from build123d import *

# Parameters (mm, degrees)
SKETCH1_R           = 19
SKETCH1_R_2         = 1
BOSS_EXTRUDE1_DEPTH = 1.6
SKETCH2_W           = 16.970562748
SKETCH2_H           = 3.563360777
SKETCH2_W_2         = 5.149879678
SKETCH2_H_2         = 16.970562749
CUT_EXTRUDE1_DEPTH  = 1.6
CUT_EXTRUDE2_DEPTH  = 1.6
SKETCH4_W           = 16
SKETCH4_H           = 11.067837439
CUT_EXTRUDE3_DEPTH  = 1.6


with BuildPart() as part:
    # Sketch1 → Boss-Extrude1 (new body)
    with BuildSketch(Plane.XY):
        with Locations((0, -13.250389013)):
            Circle(SKETCH1_R)
        with Locations((-10, -3.250389013)):
            Circle(SKETCH1_R_2, mode=Mode.SUBTRACT)
        with Locations((10, -3.250389013)):
            Circle(SKETCH1_R_2, mode=Mode.SUBTRACT)
        with Locations((10, -23.250389013)):
            Circle(SKETCH1_R_2, mode=Mode.SUBTRACT)
        with Locations((-10, -23.250389013)):
            Circle(SKETCH1_R_2, mode=Mode.SUBTRACT)
    extrude(amount=BOSS_EXTRUDE1_DEPTH)

    # Sketch2 → Cut-Extrude1 (cut)
    with BuildSketch(Plane.XY.offset(1.6)):
        with Locations((0, 5.531291376)):
            Rectangle(SKETCH2_W, SKETCH2_H)
        with Locations((-19.574939839, -13.250389013)):
            Rectangle(SKETCH2_W_2, SKETCH2_H_2)
    extrude(amount=-CUT_EXTRUDE1_DEPTH, mode=Mode.SUBTRACT)

    # Sketch3 → Cut-Extrude2 (cut)
    with BuildSketch(Plane(origin=(0, 0, 0), x_dir=(-1, 0, 0), z_dir=(0, 0, -1))):
        Polygon((12.5, -5.150389013), (12.5, -7.050389013), (17, -7.050389013), (24.21815824, -7.050389013), (24.21815824, 1.058699009), (18.989854596, 1.058699009), (12.5, 1.058699009), align=None)
    cut_extrude2 = extrude(amount=-CUT_EXTRUDE2_DEPTH, mode=Mode.SUBTRACT)

    # Mirror1: Cut-Extrude2 across plane
    add(cut_extrude2.mirror(Plane(origin=(0, 0, 0), x_dir=(0, 0, 1), z_dir=(1, 0, 0))), mode=Mode.SUBTRACT)

    # Sketch4 → Cut-Extrude3 (cut)
    with BuildSketch(Plane.XY.offset(1.6)):
        with Locations((0, -31.284307733)):
            Rectangle(SKETCH4_W, SKETCH4_H)
    extrude(amount=-CUT_EXTRUDE3_DEPTH, mode=Mode.SUBTRACT)


solid = part.part
Here's how the part is built. I have some questions about the finished solid (model axes, mm). A direction names the side the tool comes from. Coordinates: 2 decimals unless noted, no trailing zeros. Order: outer loops, then holes, each group sorted by start corner. A loop starts at its lowest first (then second) coordinate and runs counter-clockwise, first axis right, second up.
Item 1: For P1, Ø0.5, axis at y = -27.5, z = 1, coming from the -X side, with a flat end and sliding along its axis, tell me the tip position at first contact or that it passes through.
Result sheet:
P1: stops at x = -12.85
Item 2: I need wall thicknesses on line 1 (Y direction, x = 10, z = 1.1); line 2 (X direction, y = -4, z = 0.2); line 3 (Y direction, x = -6, z = 1.4). Which ranges of each line are inside material? Lowest first, please.
Result sheet:
line 1: y = -29.41 to -24.25, -22.25 to -4.25, -2.25 to 2.91
line 2: x = -12.5 to -10.66, -9.34 to 9.34, 10.66 to 12.5
line 3: y = -25.75 to 3.75
Item 3: If we section it at A-A on x = 10: List the corners of the cut face in (y, z) for me, plus the area to 3 significant figures.
Result sheet:
outline: (-29.41, 0) - (-24.25, 0) - (-24.25, 1.6) - (-29.41, 1.6) - close; (-22.25, 0) - (-4.25, 0) - (-4.25, 1.6) - (-22.25, 1.6) - close; (-2.25, 0) - (2.91, 0) - (2.91, 1.6) - (-2.25, 1.6) - close
area: 45.3 mm2
Item 4: For faces 5 (the face through (12.5, -3, 1)), 6 (the face through (-17, -14, 1)), 7 (the face through (8, -28, 1)), 8 (the face through (0, 3.75, 1)), 9 (the face through (-15, -7.05, 1)), which set-ups out of +Z, -Z, +X, -X, +Y, -Y let a thin tool reach every point of the face, with its end or its side?
Result sheet:
face 5: +Z, -Z, +X, +Y
face 6: +Z, -Z, -X, +Y, -Y
face 7: +Z, -Z, -Y
face 8: +Z, -Z, +X, -X, +Y
face 9: +Z, -Z, -X, +Y
Item 5: If we section it at C-C on x = 3.5: List the corners of the cut face in (y, z) for me, plus the area to 3 significant figures.
Result sheet:
outline: (-25.75, 0) - (3.75, 0) - (3.75, 1.6) - (-25.75, 1.6) - close
area: 47.2 mm2
Item 6: If we section it at D-D on y = -1: List the corners of the cut face in (x, z) for me, plus the area to 3 significant figures.
Result sheet:
outline: (-12.5, 0) - (12.5, 0) - (12.5, 1.6) - (-12.5, 1.6) - close
area: 40.0 mm2
Item 7: If we mould it in two halves opening along X, with no side actions, what happens to faces 1 (the face through (15, -7.05, 1)), 2 (the face through (-10.794, -3.859, 0.789)), 3 (the face through (0, -25.75, 1)), 4 (the face through (17.41, -20.86, 0.79))? For each: +X half, -X half, draft (parallel to the pull), parting line (faces both ways), or undercut.
Result sheet:
face 1: draft
face 2: undercut
face 3: undercut
face 4: +X half
Item 8: If we section it at B-B on z = 1.25: List the corners of the cut face in (x, y) for me, plus the area to 3 significant figures.
Result sheet:
outline: (-17, -21.74) arc R19 ccw to (-8, -30.48) - (-8, -25.75) - (8, -25.75) - (8, -30.48) arc R19 ccw to (17.96, -7.05) - (12.5, -7.05) - (12.5, 1.06) arc R19 ccw to (8.49, 3.75) - (-8.49, 3.75) arc R19 ccw to (-12.5, 1.06) - (-12.5, -7.05) - (-17, -7.05) - close; hole circle Ø2 at (-10, -23.25); hole circle Ø2 at (-10, -3.25); hole circle Ø2 at (10, -23.25); hole circle Ø2 at (10, -3.25)
area: 930 mm2
